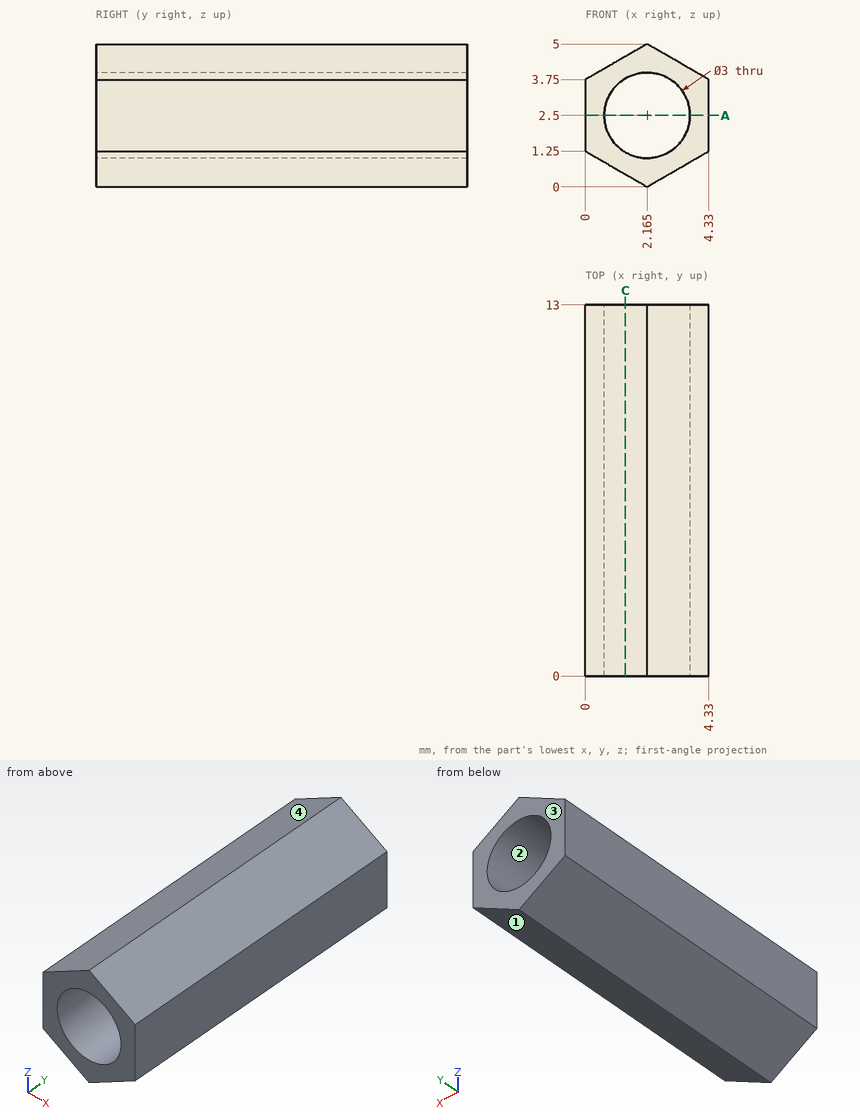
For this review, use the dimensioned drawing (mm, ordinates from the lowest corner) and the shaded views. Give positions to 0.01 mm unless a question says otherwise; leave off trailing zeros. Order: outer loops, then holes, each group sorted by start corner. A loop starts at its lowest first (then second) coordinate and runs counter-clockwise, first axis right, second up.
1. To check wall thickness, follow L1, parallel to Z at x = 3.25, y = 5.25 (1 decimal); L2, parallel to Z at x = 2.3, y = 11.5; L3, parallel to X at y = 6.75, z = 2.7. State the ranges of each line that lie inside material, in increasing order.
Solution:
L1: z = 0.6 to 1.5, 3.5 to 4.4
L2: z = 0.08 to 1.01, 3.99 to 4.92
L3: x = 0 to 0.68, 3.65 to 4.33
2. Mouldability with a two-part tool opening along Z and no side actions: class the marked faces 1, 2, 3 and 4 as +Z half, -Z half, draft (parallel to the pull), parting line (faces both ways), or undercut.
Solution:
face 1: -Z half
face 2: undercut
face 3: draft
face 4: +Z half
3. Add section A-A, the plane z = 2.5. State the section outline as (x, y) points (1 decimal), then the cut area to 3 significant figures.
Solution:
outline: (0, 0) - (0.7, 0) - (0.7, 13) - (0, 13) - close; (3.7, 0) - (4.3, 0) - (4.3, 13) - (3.7, 13) - close
area: 17.3 mm2
4. Add section C-C, the plane x = 1.4. State the section outline as (y, z) points.
Solution:
outline: (0, 0.44) - (13, 0.44) - (13, 1.21) - (0, 1.21) - close; (0, 3.79) - (13, 3.79) - (13, 4.56) - (0, 4.56) - close
5. For pin 1 Ø1.5 at (x, y) = (3, 9) entering from -Z; pin 2 Ø1 at (y, z) = (11, 4.5) entering from -X, all flat-tipped, find the tip position at first contact; note any pin that passes through.
Solution:
pin 1: stops at z = 0.05
pin 2: stops at x = 0.43
